For this review, take the finished solid that the model builds, in its own axes (mm). Face numbers are marked on the shaded views. Give positions to 0.01 mm unless a question says otherwise; leave off trailing zeros. Loops run counter-clockwise (first coordinate to the right, second up) from the corner with the lowest first, then second, coordinate; pieces in that order, holes last.
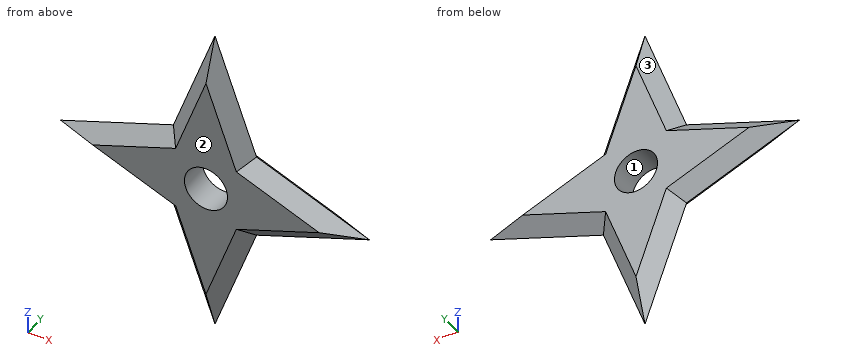
```python
from build123d import *

# Parameters (mm, degrees)
F1_DEPTH = 10.16
F2_SIZE  = 5.07999
F4_D     = 15.24


# Not quite as in the source:
# - a fillet or chamfer is up to 0.001 mm smaller than in the source, because OpenCascade refuses the exact size


with BuildPart() as f1:
    # F0 (on Front) → F1 (new body)
    with BuildSketch(Plane.XZ):
        Polygon((14.7110316902, 14.8611441255), (0, 54.7910891473), (-14.7110316902, 14.8611441255), (0, 0), align=None)
        Polygon((54.6409785748, 0), (14.7110316902, 14.8611441255), (0, 0), (14.7110316902, -14.8611441255), align=None)
        Polygon((14.7110316902, -14.8611441255), (0, 0), (-14.7110316902, -14.8611441255), (0, -54.7910891473), align=None)
        Polygon((0, 0), (-14.7110316902, 14.8611441255), (-54.6409785748, 0), (-14.7110316902, -14.8611441255), align=None)
    extrude(amount=F1_DEPTH)

    # F2 (size 5.08 in the source; OpenCascade refuses exactly that, so slightly less here)
    f2_edges = [f1.edges().sort_by_distance(p)[0] for p in [
        (7.355516, 0, 34.826117),
        (-7.355516, 0, 34.826117),
        (-7.355516, -10.16, 34.826117),
        (7.355516, -10.16, 34.826117),
        (-34.676005, -10.16, 7.430572),
        (-34.676005, 0, 7.430572),
        (-34.676005, -10.16, -7.430572),
        (-34.676005, 0, -7.430572),
        (34.676005, 0, -7.430572),
        (34.676005, 0, 7.430572),
        (34.676005, -10.16, 7.430572),
        (34.676005, -10.16, -7.430572),
        (-7.355516, 0, -34.826117),
        (7.355516, 0, -34.826117),
        (-7.355516, -10.16, -34.826117),
        (7.355516, -10.16, -34.826117),
    ]]
    chamfer(f2_edges, length=F2_SIZE)

    # F4 (through all)
    with Locations(Plane(origin=(0, 0, 0), x_dir=(1, 0, 0), z_dir=(0, 1, 0))):
        with Locations((0, 0)):
            Hole(F4_D / 2)


solid = f1.part
```
Q1. Mouldability with a two-part tool opening along X and no side actions: class the marked faces 1, 2 and 3 as +X half, -X half, draft (parallel to the pull), parting line (faces both ways), or undercut.
Answers:
face 1: undercut
face 2: draft
face 3: -X half
Q2. For pin 1 Ø2 at (y, z) = (-7, 40.5) entering from -X; pin 2 Ø1.5 at (x, z) = (-23.5, 9.5) entering from +Y; pin 3 Ø6 at (x, y) = (-22.5, -9) entering from +Z, all flat-tipped, find the tip position at first contact; note any pin that passes through.
Answers:
pin 1: stops at x = -4.35
pin 2: stops at y = -2.37
pin 3: stops at z = 11.17
Q3. For probe 1 along Y at (x, z) = (23, -10); probe 2 along Z at (x, y) = (33.5, -3.25); probe 3 along Z at (x, y) = (17, -8.5), list the stretches that pass through material, from the lowest coordinate up.
Answers:
probe 1: y = -6.74 to -3.42
probe 2: z = -5.92 to 5.92
probe 3: z = -10.36 to 10.36
Q4. Consider section A-A on y = -7.25. Give the boundary of the cut face in (x, z).
Answers:
outline: (-48.42, 0) - (-13.02, -13.18) - (0, -48.51) - (13.02, -13.18) - (48.42, 0) - (13.02, 13.18) - (0, 48.51) - (-13.02, 13.18) - close; hole circle Ø15.24 at (0, 0)
